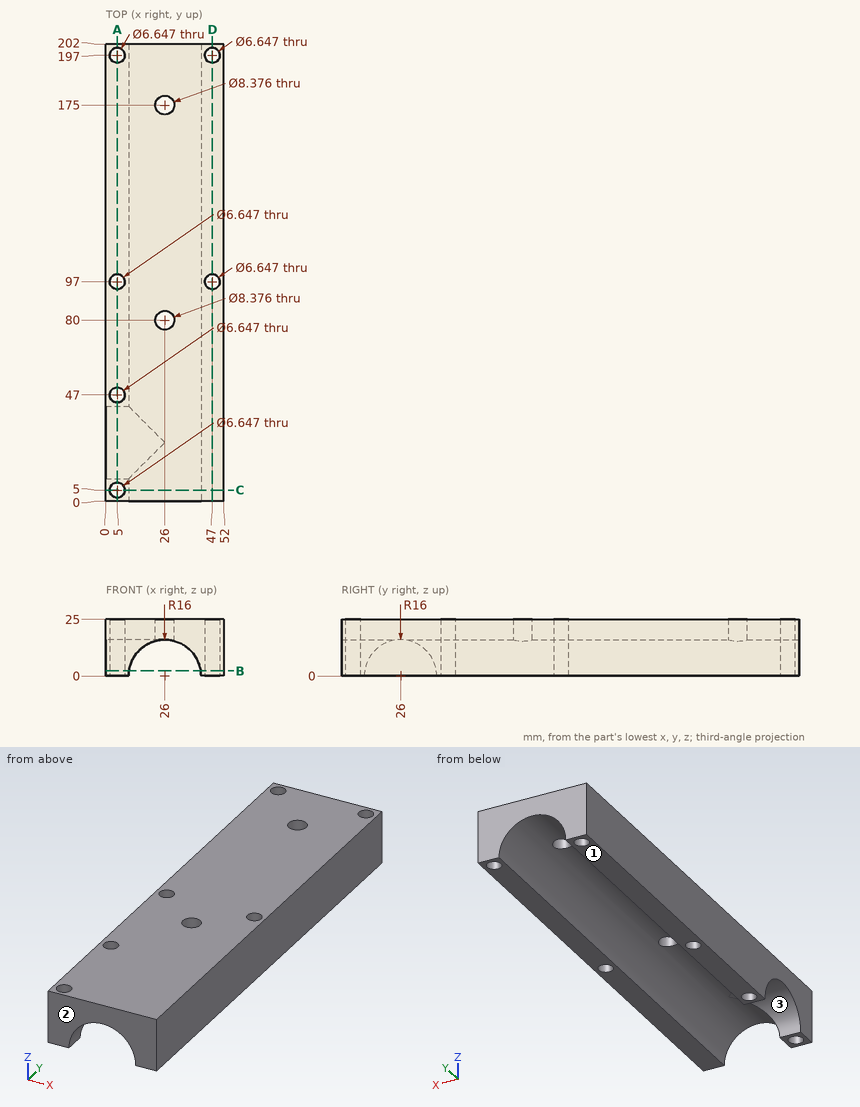
For this review, use the dimensioned drawing (mm, ordinates from the lowest corner) and the shaded views. Round coordinates to 2 decimals unless told otherwise and drop trailing zeros. Write each loop counter-clockwise with the first axis right and the second up, starting at its lowest first coordinate (ties: lowest second). Pieces come first, ordered by that corner, then holes. Notation, with made-up numbers: (-18, 23) -> (6, 23) arc R16 ccw to (6, 33) -> close; hole circle Ø8 at (56.25, 18.25). An arc over 180 degrees is marked (long way). Use CSV: the item, a comma, the result in double quotes.
(1) Consider section B-B, the plane z = 2.25. Give the number of separate pieces and of enclosed holes in the cut face, plus the area to 3 significant figures.
Computed values:
separate pieces,"3"
enclosed holes,"6"
area,"3,570 mm²"
(2) Clearance check with flat-ended pins moving along their axes: P1, Ø6, axis at x = 5, y = 97, coming from the +Z side; P2, Ø13.5, axis at x = 26, y = 175, coming from the -Z side. State where each tip first meets the part, or that it passes through.
Computed values:
P1,"through"
P2,"z = 14.51"
(3) Consider section A-A, the plane x = 5. Give the boundary of the cut face in (y, z).
Computed values:
outline,"(0, 0) -> (1.68, 0) -> (1.68, 25) -> (0, 25) -> close; (8.32, 0) -> (10, 0) arc R16 cw to (42, 0) -> (43.68, 0) -> (43.68, 25) -> (8.32, 25) -> close; (50.32, 0) -> (93.68, 0) -> (93.68, 25) -> (50.32, 25) -> close; (100.32, 0) -> (193.68, 0) -> (193.68, 25) -> (100.32, 25) -> close; (200.32, 0) -> (202, 0) -> (202, 25) -> (200.32, 25) -> close"
(4) Consider section D-D, the plane x = 47. Give the boundary of the cut face in (y, z), plus the area to 3 significant figures.
Computed values:
outline,"(0, 0) -> (93.68, 0) -> (93.68, 25) -> (0, 25) -> close; (100.32, 0) -> (193.68, 0) -> (193.68, 25) -> (100.32, 25) -> close; (200.32, 0) -> (202, 0) -> (202, 25) -> (200.32, 25) -> close"
area,"4,720 mm²"
(5) Draft analysis for pull direction Y (two halves, no side actions). For the marked faces 1, 2 and 3, state which applies: +Y half, -Y half, draft (parallel to the pull), parting line (faces both ways), or undercut.
Computed values:
face 1,"draft"
face 2,"-Y half"
face 3,"undercut"
(6) Consider section C-C, the plane y = 5. Give the boundary of the cut face in (x, z), plus the area to 3 significant figures.
Computed values:
outline,"(0, 0) -> (1.68, 0) -> (1.68, 25) -> (0, 25) -> close; (8.32, 0) -> (10, 0) arc R16 cw to (42, 0) -> (52, 0) -> (52, 25) -> (8.32, 25) -> close"
area,"732 mm²"
(7) To check wall thickness, follow L1, parallel to Y at x = 47, z = 15.75; L2, parallel to X at y = 197, z = 18; L3, parallel to Y at x = 26, z = 19.25. State the ranges of each line that lie inside material, in increasing order. Write a range as [from, to].
Computed values:
L1,"[0, 93.68], [100.32, 193.68], [200.32, 202]"
L2,"[0, 1.68], [8.32, 43.68], [50.32, 52]"
L3,"[0, 75.81], [84.19, 170.81], [179.19, 202]"
